Design review of the part built by this model. Coordinates are the model's own, in mm. Face numbers are marked on the shaded views. A direction names the side the tool comes from. Coordinates: 2 decimals unless noted, no trailing zeros. Loops run counter-clockwise (first coordinate to the right, second up) from the corner with the lowest first, then second, coordinate; pieces in that order, holes last.
Q1. Machinability: for the marked faces 1, 2, 3, 4 and 5, which of the approach directions +Z, -Z, +X, -X, +Y, -Y give a long, thin tool a straight path to every point of the face, cutting with its end or side? Answer none if there is none.
Q2. Wall thickness on probe 1 along Y at (x, z) = (-5.75, 5); probe 2 along Z at (x, y) = (4.5, 3.5); probe 3 along Z at (x, y) = (-2, -4): over which ranges is each line inside the solid? List them lowest first.
Q3. Add section A-A on y = -4. Give the boundary of the cut face in (x, z), and give its area (3 significant figures).
Q4. Add section C-C on x = 4.5. Give the boundary of the cut face in (y, z), and give its area (3 significant figures).
Q5. Draft analysis for pull direction X (two halves, no side actions). For the marked faces 6, 7 and 8, state which applies: released by +X, released by -X, zero draft, split by the parting line, or undercut.
Q6. Add section B-B on z = 3. Give the boundary of the cut face in (x, y).
Q7. Add section D-D on y = -1.75. Give the boundary of the cut face in (x, z), and give its area (3 significant figures).
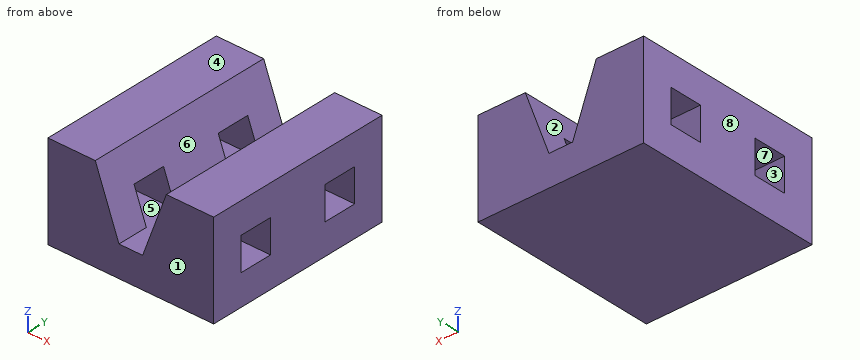
```python
from build123d import *

# Parameters (mm, degrees)
ESBO_O1_W                = 14
ESBO_O1_H                = 16
RESSALTO_EXTRUS_O1_DEPTH = 8
ESBO_O3_W                = 2.8
ESBO_O3_H                = 2.8
CORTE_EXTRUS_O2_DEPTH    = 19
CORTE_EXTRUS_O3_DEPTH    = 20.209372712


with BuildPart() as part:
    # Esbo_o1 → Ressalto-extrus_o1 (new body)
    with BuildSketch(Plane.XY):
        Rectangle(ESBO_O1_W, ESBO_O1_H)
    extrude(amount=RESSALTO_EXTRUS_O1_DEPTH)

    # Esbo_o3 → Corte-extrus_o2 (cut, through all)
    with BuildSketch(Plane(origin=(7, 0, 0), x_dir=(0, 0, -1), z_dir=(1, 0, 0))):
        with Locations((-4, 4)):
            Rectangle(ESBO_O3_W, ESBO_O3_H)
        with Locations((-4, -4)):
            Rectangle(ESBO_O3_W, ESBO_O3_H)
    extrude(amount=-CORTE_EXTRUS_O2_DEPTH, mode=Mode.SUBTRACT)

    # Esbo_o5 → Corte-extrus_o3 (cut, through all)
    with BuildSketch(Plane(origin=(0, 8, 0), x_dir=(1, 0, 0), z_dir=(0, 1, 0))):
        Polygon((1, -2.6), (0, -2.6), (0, -8), (3, -8), align=None)
        Polygon((0, -2.6), (-1, -2.6), (-3, -8), (0, -8), align=None)
    extrude(amount=-CORTE_EXTRUS_O3_DEPTH, mode=Mode.SUBTRACT)


solid = part.part
```
Entries:
1. face 1: +Z, -Z, +X, -X, -Y
1. face 2: +Z, +Y, -Y
1. face 3: +X, -X
1. face 4: +Z, +X, -X, +Y, -Y
1. face 5: none
2. probe 1: y = -8 to -5.4, -2.6 to 2.6, 5.4 to 8
2. probe 2: z = 0 to 2.6, 5.4 to 8
2. probe 3: z = 0 to 2.6
3. outline: (-7, 0) - (7, 0) - (7, 2.6) - (-7, 2.6) - close; (-7, 5.4) - (-2.04, 5.4) - (-3, 8) - (-7, 8) - close; (2.04, 5.4) - (7, 5.4) - (7, 8) - (3, 8) - close
3. area: 59.7 mm2
4. outline: (-8, 0) - (8, 0) - (8, 8) - (-8, 8) - close; hole (-5.4, 2.6) - (-2.6, 2.6) - (-2.6, 5.4) - (-5.4, 5.4) - close; hole (2.6, 2.6) - (5.4, 2.6) - (5.4, 5.4) - (2.6, 5.4) - close
4. area: 112 mm2
5. face 6: undercut
5. face 7: zero draft
5. face 8: released by -X
6. outline: (-7, -8) - (-1.15, -8) - (-1.15, -5.4) - (-7, -5.4) - close; (-7, -2.6) - (-1.15, -2.6) - (-1.15, 2.6) - (-7, 2.6) - close; (-7, 5.4) - (-1.15, 5.4) - (-1.15, 8) - (-7, 8) - close; (1.15, -8) - (7, -8) - (7, -5.4) - (1.15, -5.4) - close; (1.15, -2.6) - (7, -2.6) - (7, 2.6) - (1.15, 2.6) - close; (1.15, 5.4) - (7, 5.4) - (7, 8) - (1.15, 8) - close
7. outline: (-7, 0) - (7, 0) - (7, 8) - (3, 8) - (1, 2.6) - (-1, 2.6) - (-3, 8) - (-7, 8) - close
7. area: 90.4 mm2
